```python
from build123d import *

# Parameters (mm, degrees)
BOSS_EXTRU_1_DEPTH      = 5
ENL_V_MAT_EXTRU_1_DEPTH = 5
ENL_V_MAT_EXTRU_2_DEPTH = 5
SYM_TRIE2_COPY_1_DEPTH  = 5
ENL_V_MAT_EXTRU_3_DEPTH = 10


with BuildPart() as part:
    # Esquisse1 → Boss.-Extru.1 (new body)
    with BuildSketch(Plane(origin=(0, 0, 0), x_dir=(1, 0, 0), z_dir=(0, 1, 0))):
        Polygon((17.5, -5), (37.5, -5), (37.5, 0), (55, 0), (55, -60), (55, -65), (37.5, -65), (37.5, -60), (17.5, -60), (17.5, -65), (0, -65), (0, -60), (0, -42.5), (-5, -42.5), (-5, -22.5), (0, -22.5), (0, 0), (17.5, 0), align=None)
    extrude(amount=BOSS_EXTRU_1_DEPTH)

    # Esquisse2 → Enlèv. mat.-Extru.1 (cut)
    with BuildSketch(Plane(origin=(0, 5, 0), x_dir=(1, 0, 0), z_dir=(0, 1, 0))):
        with BuildLine():
            Line((25, -21), (30, -21))
            ThreePointArc((30, -21), (41.5, -32.5), (30, -44))
            Line((30, -44), (25, -44))
            ThreePointArc((25, -44), (13.5, -32.5), (25, -21))
        make_face()
    extrude(amount=-ENL_V_MAT_EXTRU_1_DEPTH, mode=Mode.SUBTRACT)

    # Esquisse3 → Enlèv. mat.-Extru.2 (cut)
    with BuildSketch(Plane(origin=(0, 5, 0), x_dir=(1, 0, 0), z_dir=(0, 1, 0))):
        with BuildLine():
            Line((9.5, -15), (14.5, -15))
            ThreePointArc((14.5, -15), (16.5, -17), (14.5, -19))
            Line((14.5, -19), (9.5, -19))
            ThreePointArc((9.5, -19), (7.5, -17), (9.5, -15))
        make_face()
    enl_v_mat_extru_2 = extrude(amount=-ENL_V_MAT_EXTRU_2_DEPTH, mode=Mode.SUBTRACT)

    # Symétrie1: Enlèv. mat.-Extru.2 across plane
    add(enl_v_mat_extru_2.mirror(Plane.XY.offset(32.5)), mode=Mode.SUBTRACT)

    # Symétrie2: Enlèv. mat.-Extru.2 across plane
    add(enl_v_mat_extru_2.mirror(Plane.ZY.offset(-27.5)), mode=Mode.SUBTRACT)

    # Symétrie2 copy 1 sketch → Symétrie2 copy 1 (cut)
    with BuildSketch(Plane(origin=(55, 5, 65), x_dir=(-1, 0, 0), z_dir=(0, 1, 0))):
        with BuildLine():
            Line((9.5, -15), (14.5, -15))
            ThreePointArc((14.5, -15), (16.5, -17), (14.5, -19))
            Line((14.5, -19), (9.5, -19))
            ThreePointArc((9.5, -19), (7.5, -17), (9.5, -15))
        make_face()
    extrude(amount=-SYM_TRIE2_COPY_1_DEPTH, mode=Mode.SUBTRACT)

    # Esquisse4 → Enlèv. mat.-Extru.3 (cut)
    with BuildSketch(Plane(origin=(0, 5, 0), x_dir=(1, 0, 0), z_dir=(0, 1, 0))):
        Polygon((13, -5.9), (11, -5.9), (11, -4.75), (8.5, -4.75), (8.5, -5.9), (0, -5.9), (0, -9.1), (8.5, -9.1), (8.5, -10.25), (11, -10.25), (11, -9.1), (13, -9.1), align=None)
    enl_v_mat_extru_3 = extrude(amount=-ENL_V_MAT_EXTRU_3_DEPTH, mode=Mode.SUBTRACT)

    # Symétrie3: Enlèv. mat.-Extru.3 across plane
    add(enl_v_mat_extru_3.mirror(Plane.XY.offset(32.5)), mode=Mode.SUBTRACT)


solid = part.part
```
Source: CAD feature listing. Evaluate the final solid. Frame: model axes, mm. A direction names the side the tool comes from. Round coordinates to 2 decimals unless told otherwise and drop trailing zeros. Write each loop counter-clockwise with the first axis right and the second up, starting at its lowest first coordinate (ties: lowest second). Pieces come first, ordered by that corner, then holes. Notation, with made-up numbers: M 38,42.25 L 58,42.25 A12 ccw 58,48.25 Z; hole C 61.5,-30.75 d4. An arc over 180 degrees is marked long. Answer as a JSON object with one key per item and string values. Group by question number.
(1) First-contact query: pin 1 (2.5 mm diameter, centred on y = 1.5, z = 2.5, fed in from -X); pin 2 (10 mm diameter, centred on x = 29.5, z = 26.5, fed in from +Y); pin 3 (2.5 mm diameter, centred on x = 27.5, y = 3.5, fed in from -Z); pin 4 (2.5 mm diameter, centred on x = -2, y = 3, fed in from -Z). Flat tips, straight axial feed; report the tip coordinate or a pass-through.
(2) Mould query, pull axis Z, two halves, no side actions, for faces 6 (the flat face through (9, 2, 65)), 7 (the flat face through (13, 3, 57)), 8 (the flat face through (37.5, 2, 3)). Classes: +Z half, -Z half, draft (parallel to the pull), parting line (faces both ways), or undercut.
(3) Section query C-C on z = 32.5. Output: boundary loops of the cut face in (x, y).
(4) Section query D-D on y = 1.2. State how many separate pieces and enclosed holes the cut face has, then the cut area to 3 significant figures.
(5) Section query B-B on x = 5. Output: boundary loops of the cut face in (y, z).
(6) Reachability of faces 1 (the flat face through (28, 2, 60)), 2 (the flat face through (4, 3, 59.1)), 3 (the flat face through (-2, 2, 42.5)), 4 (the flat face through (17.5, 2, 2)), 5 (the cylindrical face through (16.5, 2.5, 48)) from +Z, -Z, +X, -X, +Y, -Y: full face, straight path, thin tool, end or side. Return the list, or none.
(7) Section query A-A on z = 17. Output: boundary loops of the cut face in (x, y), then the cut area to 3 significant figures.
(8) Ray query, line 1 (Z direction, x = 10, y = 0.6); line 2 (X direction, y = 3.95, z = 47); line 3 (X direction, y = 2.5, z = 62.5). Return the intervals inside material, ascending. Write a range as [from, to].
Computed values:
{
 "1": {"pin 1": "x = 0", "pin 2": "through", "pin 3": "z = 5", "pin 4": "z = 22.5"},
 "2": {"face 6": "+Z half", "face 7": "undercut", "face 8": "draft"},
 "3": {"outline": "M -5,0 L 13.5,0 L 13.5,5 L -5,5 Z; M 41.5,0 L 55,0 L 55,5 L 41.5,5 Z"},
 "4": {"separate pieces": "1", "enclosed holes": "5", "area": "2,720 mm^2"},
 "5": {"outline": "M 0,0 L 5,0 L 5,5.9 L 0,5.9 Z; M 0,9.1 L 5,9.1 L 5,55.9 L 0,55.9 Z; M 0,59.1 L 5,59.1 L 5,65 L 0,65 Z"},
 "6": {"face 1": "+Z, +Y, -Y", "face 2": "-X, +Y, -Y", "face 3": "+Z, -X, +Y, -Y", "face 4": "-Z, +Y, -Y", "face 5": "+Y, -Y"},
 "7": {"outline": "M 0,0 L 7.5,0 L 7.5,5 L 0,5 Z; M 16.5,0 L 38.5,0 L 38.5,5 L 16.5,5 Z; M 47.5,0 L 55,0 L 55,5 L 47.5,5 Z", "area": "185 mm^2"},
 "8": {"line 1": "[0, 4.75], [10.25, 15], [19, 46], [50, 54.75], [60.25, 65]", "line 2": "[0, 7.77], [16.23, 38.77], [47.23, 55]", "line 3": "[0, 17.5], [37.5, 55]"}
}
